Read the model definition and answer for the solid it produces. Units are mm, in the model's axes. A direction names the side the tool comes from. Round coordinates to 2 decimals unless told otherwise and drop trailing zeros. Order: outer loops, then holes, each group sorted by start corner. A loop starts at its lowest first (then second) coordinate and runs counter-clockwise, first axis right, second up. Notation, with made-up numbers: (-34, 66.25) - (9, 66.25) arc R28 ccw to (9, 103.25) - close; hole circle Ø7 at (87.25, -3.5). An arc over 180 degrees is marked (long way). One line per question, with ' | ' between items. Start each with the question number.
1) For faces 5 (the flat face through (0, 0, -35)), 6 (the flat face through (1.25, 0, 2)), 7 (the cylindrical face through (-1.43, -0.32, -17.74)), determine the directions among +Z, -Z, +X, -X, +Y, -Y from which every point of the face is accessible in a straight line to the end or side of a thin tool.
2) Flat-ended cylindrical pins translate along their axes: pin 1 (1.5 mm diameter, centred on x = 0, z = -29.5, fed in from +Y) (3 decimals); pin 2 (2 mm diameter, centred on x = -2, z = -1.5, fed in from -Y); pin 3 (3 mm diameter, centred on y = 1, z = -12.5, fed in from +X) (3 decimals). Find the tip coordinate at first contact, or state that the pin passes through.
3) Straight lines are drawn through the part: line 1 (Z direction, x = 0, y = -0.2); line 2 (Z direction, x = -1.7, y = 1.6); line 3 (X direction, y = 0.45, z = 1.5). For each, find the intervals that lie inside material, in ascending order. Write a range as from..to.
4) The part is cut by section B-B, the plane z = -27. Give the vertices of the cut face in (x, y) (3 decimals).
5) The mould has two halves that part along X. Classify faces 1 (the flat face through (0.63, 1.08, 2.16)), 2 (the cylindrical face through (-2.685, -0.596, 1.482)), 3 (the flat face through (-1.1, -1.1, 3)), 4 (the flat face through (-1.25, 0, 2)): pulls with the +X half, pulls with the -X half, needs draft (parallel to the pull), parting line crosses it, or undercut.
6) The part is cut by section A-A, the plane y = 0. Give the vertices of the cut face in (x, z) (3 decimals).
from build123d import *

# Parameters (mm, degrees)
SCHNITT_LINEAR_AUSTRAGEN1_DEPTH = 1.8
FASE1_SIZE                      = 0.2
VERRUNDUNG1_R                   = 0.2
VERRUNDUNG2_R                   = 0.1


with BuildPart() as part:
    # Skizze1 → Rotation1 (revolve)
    with BuildSketch(Plane(origin=(0, 0, 0), x_dir=(0, 0, -1), z_dir=(1, 0, 0))):
        Polygon((-3, 0), (-3, 2.75), (0, 2.75), (0, 1.465), (35, 1.465), (35, 0), align=None)
    revolve(axis=Axis((0, 0, 21.919879518), (0, 0, -1)))

    # Skizze2 → Schnitt-Linear austragen1 (cut)
    with BuildSketch(Plane.XY.offset(3)):
        Polygon((1.25, -0.721687836), (1.25, 0.721687836), (0, 1.443375673), (-1.25, 0.721687836), (-1.25, -0.721687836), (0, -1.443375673), align=None)
    extrude(amount=-SCHNITT_LINEAR_AUSTRAGEN1_DEPTH, mode=Mode.SUBTRACT)

    # Fase1
    fase1_edges = [part.edges().sort_by_distance(p)[0] for p in [
        (0, -1.465, -35),
        (0, -2.75, 0),
        (0, -2.75, 3),
    ]]
    chamfer(fase1_edges, length=FASE1_SIZE)

    # Verrundung1
    verrundung1_edges = [part.edges().sort_by_distance(p)[0] for p in [
        (0.625, -1.082531755, 1.2),
        (1.25, -0.721687836, 2.1),
        (-0.625, -1.082531755, 1.2),
        (0, -1.443375673, 2.1),
        (-1.25, 0, 1.2),
        (-1.25, -0.721687836, 2.1),
        (-0.625, 1.082531755, 1.2),
        (-1.25, 0.721687836, 2.1),
        (0.625, 1.082531755, 1.2),
        (0, 1.443375673, 2.1),
        (1.25, 0, 1.2),
        (1.25, 0.721687836, 2.1),
        (0, -1.465, 0),
    ]]
    fillet(verrundung1_edges, radius=VERRUNDUNG1_R)

    # Verrundung2
    verrundung2_edges = [part.edges().sort_by_distance(p)[0] for p in [
        (-0.625, -1.082531755, 3),
        (-1.25, 0, 3),
        (-0.625, 1.082531755, 3),
        (0.625, 1.082531755, 3),
        (1.25, 0, 3),
        (0.625, -1.082531755, 3),
        (-1.223205081, -0.706217783, 3),
        (0, -1.412435565, 3),
        (1.223205081, -0.706217783, 3),
        (1.223205081, 0.706217783, 3),
        (0, 1.412435565, 3),
        (-1.223205081, 0.706217783, 3),
    ]]
    fillet(verrundung2_edges, radius=VERRUNDUNG2_R)


solid = part.part
Values:
1) face 5: -Z, +X, -X, +Y, -Y | face 6: +Z | face 7: -Z
2) pin 1: stops at y = 1.465 | pin 2: stops at y = -1.07 | pin 3: stops at x = 1.465
3) line 1: z = -35..1.2 | line 2: z = 0..3 | line 3: x = -2.71..-1.25, 1.25..2.71
4) outline: circle Ø2.93 at (0, 0)
5) face 1: undercut | face 2: parting line crosses it | face 3: needs draft | face 4: undercut
6) outline: (-2.75, 0.2) - (-2.55, 0) - (-1.665, 0) arc R0.2 cw to (-1.465, -0.2) - (-1.465, -34.8) - (-1.265, -35) - (1.265, -35) - (1.465, -34.8) - (1.465, -0.2) arc R0.2 cw to (1.665, 0) - (2.55, 0) - (2.75, 0.2) - (2.75, 2.8) - (2.55, 3) - (1.35, 3) arc R0.1 ccw to (1.25, 2.9) - (1.25, 1.4) arc R0.2 cw to (1.05, 1.2) - (-1.05, 1.2) arc R0.2 cw to (-1.25, 1.4) - (-1.25, 2.9) arc R0.1 ccw to (-1.35, 3) - (-2.55, 3) - (-2.75, 2.8) - close
